```python
from build123d import *

# Parameters (mm, degrees)
BOSS_EXTRUDE1_DEPTH        = 60
F_2_2_2_2_DIAMETER_HOLE1_D = 2.2


with BuildPart() as part:
    # Sketch1 → Boss-Extrude1 (new body)
    with BuildSketch(Plane.XY):
        with BuildLine():
            Line((-2.5, 0), (2.5, 0))
            ThreePointArc((2.5, 0), (3.95232497, 5.091230117), (7.872150073, 8.65))
            Line((7.872150073, 8.65), (7.872150073, 9.65))
            Line((7.872150073, 9.65), (-7.872150073, 9.65))
            Line((-7.872150073, 9.65), (-7.872150073, 8.65))
            ThreePointArc((-7.872150073, 8.65), (-3.95232497, 5.091230117), (-2.5, 0))
        make_face()
    extrude(amount=BOSS_EXTRUDE1_DEPTH)

    # Ø2.2 (2.2) Diameter Hole1 (through all)
    with Locations(Plane(origin=(0, 9.65, 45), x_dir=(0, 0, 1), z_dir=(0, 1, 0))):
        with Locations((0, 0), (-30, 0)):
            Hole(F_2_2_2_2_DIAMETER_HOLE1_D / 2)


solid = part.part
```
Can you work these out from the model? Positions are in its coordinate system, mm. Coordinates: 2 decimals unless noted, no trailing zeros. Loops run counter-clockwise (first coordinate to the right, second up) from the corner with the lowest first, then second, coordinate; pieces in that order, holes last. Notation, with made-up numbers: M 73.5,34 L 123.5,34 A23 ccw 123.5,69 Z; hole C 12.25,-28.75 d11. An arc over 180 degrees is marked long. Put each result on its own line as item: value. Start each with the question number.
(1) Imagine slicing it at B-B on z = 15. List the corners of the cut face in (x, y) for me.
(2) Will these pins go through, and if not, where does the flat tip stop? pin 1 Ø2 at (y, z) = (1.5, 49) entering from +X; pin 2 Ø2.5 at (x, z) = (0, 15) entering from -Y; pin 3 Ø5 at (y, z) = (1.5, 19) entering from -X.
(3) Imagine slicing it at C-C on z = 51. List the corners of the cut face in (x, y) for me.
(4) I need wall thicknesses on probe 1 along Z at (x, y) = (1, 3.25); probe 2 along X at (y, z) = (4.5, 45); probe 3 along X at (y, z) = (5, 15). Which ranges of each line are inside material? Lowest first, please.
(5) Imagine slicing it at D-D on y = 3.5. List the corners of the cut face in (x, z) for me, and give its area (3 significant figures).
(6) Imagine slicing it at A-A on x = 0. List the corners of the cut face in (y, z) for me, and give its area (3 significant figures).
Worked answers:
1. outline: M -7.87,8.65 A9.65 cw -2.5,0 L -1.1,0 L -1.1,9.65 L -7.87,9.65 Z; M 1.1,0 L 2.5,0 A9.65 cw 7.87,8.65 L 7.87,9.65 L 1.1,9.65 Z
2. pin 1: stops at x = 2.83
2. pin 2: stops at y = 0
2. pin 3: stops at x = -3.37
3. outline: M -7.87,8.65 A9.65 cw -2.5,0 L 2.5,0 A9.65 cw 7.87,8.65 L 7.87,9.65 L -7.87,9.65 Z
4. probe 1: z = 0 to 14.54, 15.46 to 44.54, 45.46 to 60
4. probe 2: x = -3.61 to -1.1, 1.1 to 3.61
4. probe 3: x = -3.9 to -1.1, 1.1 to 3.9
5. outline: M -3.16,0 L 3.16,0 L 3.16,60 L -3.16,60 Z; hole C 0,15 d2.2; hole C 0,45 d2.2
5. area: 371 mm2
6. outline: M 0,0 L 9.65,0 L 9.65,13.9 L 0,13.9 Z; M 0,16.1 L 9.65,16.1 L 9.65,43.9 L 0,43.9 Z; M 0,46.1 L 9.65,46.1 L 9.65,60 L 0,60 Z
6. area: 537 mm2
